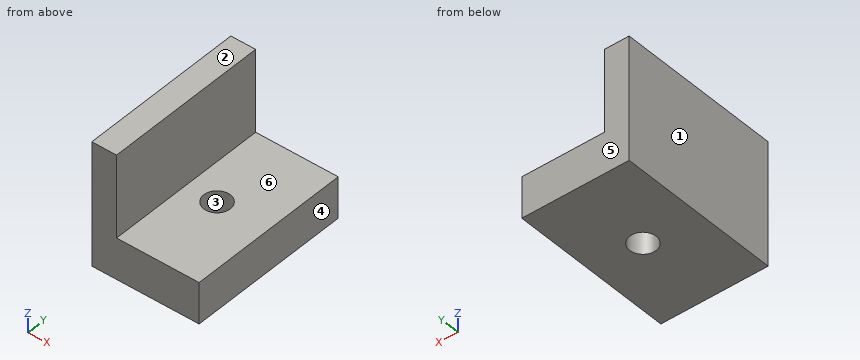
from build123d import *

# Parameters (mm, degrees)
SZKIC1_W                    = 10
SZKIC1_H                    = 20
SZKIC1_R                    = 1.6
SZKIC1_W_2                  = 3
DODANIE_WYCI_GNI_CIE1_DEPTH = 5
SZKIC2_W                    = 3
SZKIC2_H                    = 20
DODANIE_WYCI_GNI_CIE2_DEPTH = 10


with BuildPart() as part:
    # Szkic1 → Dodanie-wyciągnięcie1 (new body)
    # profile 1 of 2: a face of its own
    with BuildSketch(Plane.XY):
        with Locations((1.25, 0)):
            Rectangle(SZKIC1_W, SZKIC1_H)
        Circle(SZKIC1_R, mode=Mode.SUBTRACT)
    # profile 2 of 2: a face of its own
    with BuildSketch(Plane.XY):
        with Locations((-5.25, 0)):
            Rectangle(SZKIC1_W_2, SZKIC1_H)
    extrude(amount=DODANIE_WYCI_GNI_CIE1_DEPTH)

    # Szkic2 → Dodanie-wyciągnięcie2 (add)
    with BuildSketch(Plane.XY.offset(5)):
        with Locations((-5.25, 0)):
            Rectangle(SZKIC2_W, SZKIC2_H)
    extrude(amount=DODANIE_WYCI_GNI_CIE2_DEPTH)


solid = part.part
Geometry check sheet. Reference: the model listing, model coordinates, mm. Face numbers are marked on the shaded views. A direction names the side the tool comes from. Give positions to 0.01 mm unless a question says otherwise; leave off trailing zeros. Order: outer loops, then holes, each group sorted by start corner. A loop starts at its lowest first (then second) coordinate and runs counter-clockwise, first axis right, second up. Notation, with made-up numbers: (-28.75, -3.75) - (7.25, -3.75) arc R23 cw to (7.25, 29.25) - close; hole circle Ø10 at (-21.5, 66). An arc over 180 degrees is marked (long way). Use one line per item in the form item = value.
1) Sectioned sample at C-C (z = 3.5). Record the boundary of the cut face in (x, y).
Working result:
outline = (-6.75, -10) - (6.25, -10) - (6.25, 10) - (-6.75, 10) - close; hole circle Ø3.2 at (0, 0)
2) Sectioned sample at A-A (y = 0). Record the boundary of the cut face in (x, z), and give its area (3 significant figures).
Working result:
outline = (-6.75, 0) - (-1.6, 0) - (-1.6, 5) - (-3.75, 5) - (-3.75, 15) - (-6.75, 15) - close; (1.6, 0) - (6.25, 0) - (6.25, 5) - (1.6, 5) - close
area = 79.0 mm^2
3) Sectioned sample at B-B (x = 0). Record the boundary of the cut face in (y, z), and give its area (3 significant figures).
Working result:
outline = (-10, 0) - (-1.6, 0) - (-1.6, 5) - (-10, 5) - close; (1.6, 0) - (10, 0) - (10, 5) - (1.6, 5) - close
area = 84.0 mm^2
4) Depth check by flat-ended pin: pin 1 Ø6 at (x, y) = (4.5, -7.5) entering from +Z; pin 2 Ø3 at (x, y) = (0, 0) entering from -Z. Enter the tip coordinate at first touch or a pass-through.
Working result:
pin_1 = 5
pin_2 = through
5) Access from +Z, -Z, +X, -X, +Y, -Y to the whole of each face (thin tool, end or side, straight path). Record for the marked faces 5 and 6.
Working result:
face_5 = +Z, -Z, +X, -X, +Y
face_6 = +Z, +X, +Y, -Y
6) Sectioned sample at D-D (y = 5.5). Record the boundary of the cut face in (x, z).
Working result:
outline = (-6.75, 0) - (6.25, 0) - (6.25, 5) - (-3.75, 5) - (-3.75, 15) - (-6.75, 15) - close
7) Draft check along X on the marked faces 1, 2, 3 and 4. Enter one of: released by +X, released by -X, zero draft, split by the parting line, or undercut.
Working result:
face_1 = released by -X
face_2 = zero draft
face_3 = undercut
face_4 = released by +X
8) Material ranges on probe 1 along Y at (x, z) = (0, 3.35); probe 2 along Z at (x, y) = (-2.75, 9.25); probe 3 along X at (y, z) = (-7.5, 12), recorded low to high. Write a range as from..to.
Working result:
probe_1 = -10..-1.6, 1.6..10
probe_2 = 0..5
probe_3 = -6.75..-3.75
